```python
from build123d import *

# Parameters (mm, degrees)
BOSS_EXTRUDE1_DEPTH = 12.7
FILLET1_R           = 2.54
BOSS_EXTRUDE2_DEPTH = 15
FILLET2_R           = 1.27


with BuildPart() as part:
    # Sketch1 → Boss-Extrude1 (new body)
    with BuildSketch(Plane.XY):
        Polygon((0, 0), (0, -4.191), (-1.55575, -4.191), (-1.55575, -7.112), (0, -7.112), (0, -10.287), (10.6045, -10.287), (10.6045, -7.112), (12.16025, -7.112), (12.16025, -4.191), (10.6045, -4.191), (10.6045, 0), (18.97725, 0), (18.97725, 19.558), (15.80225, 19.558), (15.80225, 3.089), (-6.858, 3.089), (-6.858, 0), align=None)
    extrude(amount=BOSS_EXTRUDE1_DEPTH)

    # Fillet1
    fillet1_edges = [part.edges().sort_by_distance(p)[0] for p in [
        (15.80225, 3.089, 6.35),
    ]]
    fillet(fillet1_edges, radius=FILLET1_R)

    # Sketch2 → Boss-Extrude2 (add)
    with BuildSketch(Plane.XY):
        Polygon((0, 0), (0, 1.27), (10.6045, 1.27), (10.6045, 0), (10.6045, -4.191), (12.16025, -4.191), (12.16025, -7.112), (10.6045, -7.112), (10.6045, -10.287), (0, -10.287), (0, -7.112), (-1.55575, -7.112), (-1.55575, -4.191), (0, -4.191), align=None)
    extrude(amount=-BOSS_EXTRUDE2_DEPTH)

    # Fillet2
    fillet2_edges = [part.edges().sort_by_distance(p)[0] for p in [
        (5.30225, 1.27, 0),
    ]]
    fillet(fillet2_edges, radius=FILLET2_R)


solid = part.part
```
Geometry: final body of the model. Coordinates: model frame, mm. A direction names the side the tool comes from. Coordinates: 2 decimals unless noted, no trailing zeros. Order: outer loops, then holes, each group sorted by start corner. A loop starts at its lowest first (then second) coordinate and runs counter-clockwise, first axis right, second up. Notation, with made-up numbers: M 38,-17.75 L 78,-17.75 A23 cw 78,10.25 Z; hole C 32,71.25 d8. An arc over 180 degrees is marked long. Answer in a Markdown table with one row per item. Add a question column.
Q1. Mould query, pull axis Y, two halves, no side actions, for faces 1 (the flat face through (17, 19.558, 6)), 2 (the flat face through (11, -4.191, -1)), 3 (the flat face through (11, -7.112, -1)), 4 (the flat face through (7, 0, 12.7)). Classes: released by +Y, released by -Y, zero draft, split by the parting line, or undercut.
Q2. Reachability of faces 5 (the flat face through (15.802, 13, 6)), 6 (the flat face through (10.8, 2.6, 0)), 7 (the flat face through (15, 0, 6)), 8 (the flat face through (-3, 0, 6)) from +Z, -Z, +X, -X, +Y, -Y: full face, straight path, thin tool, end or side. Return the list, or none.
Q3. Section query D-D on z = 1.75. Return the cut outline in (x, y).
Q4. Line query: L1, parallel to Y at x = -1, z = 10.25; L2, parallel to Y at x = 12.5, z = 7.25; L3, parallel to Y at x = 3.75, z = 0.25. Output: solid intervals per line, ascending.
Q5. Contact query for flat-ended pins moving along their axis: P1, Ø7.5, axis at y = -0.5, z = 0, coming from the -X side; P2, Ø3, axis at x = 8, z = -9.5, coming from the +Y side; P3, Ø6, axis at x = -4, y = -1, coming from the -Z side; P4, Ø2.5, axis at x = 15.5, z = 8, coming from the -Y side. Output: stop coordinate, or through.
Q6. Section query A-A on x = 11.5. Return the cut outline in (y, z), and give its area (3 significant figures).
Q7. Section query C-C on y = 15.5. Return the cut outline in (x, z), and give its area (3 significant figures).
Q8. Section query B-B on z = -11.25. Return the cut outline in (x, y).
Completed:
| question | item | result |
|---|---|---|
| 1 | face 1 | released by +Y |
| 1 | face 2 | undercut |
| 1 | face 3 | released by -Y |
| 1 | face 4 | zero draft |
| 2 | face 5 | +Z, -Z, -X, +Y |
| 2 | face 6 | -Z, +Y |
| 2 | face 7 | +Z, -Z, +X |
| 2 | face 8 | +Z, -Z, -X |
| 3 | outline | M -6.86,0 L 0,0 L 0,-4.19 L -1.56,-4.19 L -1.56,-7.11 L 0,-7.11 L 0,-10.29 L 10.6,-10.29 L 10.6,-7.11 L 12.16,-7.11 L 12.16,-4.19 L 10.6,-4.19 L 10.6,0 L 18.98,0 L 18.98,19.56 L 15.8,19.56 L 15.8,5.63 A2.54 cw 13.26,3.09 L -6.86,3.09 Z |
| 4 | L1 | y = -7.11 to -4.19, 0 to 3.09 |
| 4 | L2 | y = 0 to 3.09 |
| 4 | L3 | y = -10.29 to 3.09 |
| 5 | P1 | stops at x = -6.86 |
| 5 | P2 | stops at y = 1.27 |
| 5 | P3 | stops at z = 0 |
| 5 | P4 | stops at y = 0 |
| 6 | outline | M -7.11,-15 L -4.19,-15 L -4.19,12.7 L -7.11,12.7 Z; M 0,0 L 3.09,0 L 3.09,12.7 L 0,12.7 Z |
| 6 | area | 120 mm2 |
| 7 | outline | M 15.8,0 L 18.98,0 L 18.98,12.7 L 15.8,12.7 Z |
| 7 | area | 40.3 mm2 |
| 8 | outline | M -1.56,-7.11 L 0,-7.11 L 0,-10.29 L 10.6,-10.29 L 10.6,-7.11 L 12.16,-7.11 L 12.16,-4.19 L 10.6,-4.19 L 10.6,1.27 L 0,1.27 L 0,-4.19 L -1.56,-4.19 Z |
